Here's the drawing with two shaded views (mm, measured from the low corner). I have some questions. A direction names the side the tool comes from. Coordinates: 2 decimals unless noted, no trailing zeros. Write each loop counter-clockwise with the first axis right and the second up, starting at its lowest first coordinate (ties: lowest second). Pieces come first, ordered by that corner, then holes. Notation, with made-up numbers: (6.25, 34) - (12.25, 34) arc R22 ccw to (12.25, 60) - close; hole circle Ø4 at (-0.5, -3). An arc over 180 degrees is marked (long way). Answer in a Markdown table with one row per item. Add a question column.
Item 1: I'm going to push flat-ended pins straight in: pin 1 (1.8 mm diameter, centred on x = 3.5, y = 5.5, fed in from -Z); pin 2 (2 mm diameter, centred on x = 4.75, y = 4.75, fed in from -Z). Where does each tip first touch, or does it pass through?
Item 2: Imagine slicing it at B-B (y = 4.75). Please give me the cut outline in (x, z) (3 decimals).
Item 3: Imagine slicing it at D-D (z = 11.75). Please give me the cut outline in (x, y) (3 decimals), plus the area to 3 significant figures.
Item 4: Imagine slicing it at A-A (x = 4.75). Please give me the cut outline in (y, z).
Item 5: Imagine slicing it at C-C (x = 67.5). Please give me the cut outline in (y, z), plus the area to 3 significant figures.
Item 6: Which directions (+Z, -Z, +X, -X, +Y, -Y) give clear straight access to the entire face, cutting with the end or side of a thin tool? Please do the marked faces 1, 2 and 3.
Item 7: If I drill on probe 1 along Y at (x, z) = (4.75, 23); probe 2 along Y at (x, z) = (4.75, 11.75); probe 3 along X at (y, z) = (43.5, 2) (3 decimals), over which ranges is the centre line in solid material (lowest first)? Write a range as from..to.
Item 8: We'd pull the mould along X, two halves only. Please class the marked faces 4, 5 and 6: +X half, -X half, draft (parallel to the pull), parting line (faces both ways), or undercut.
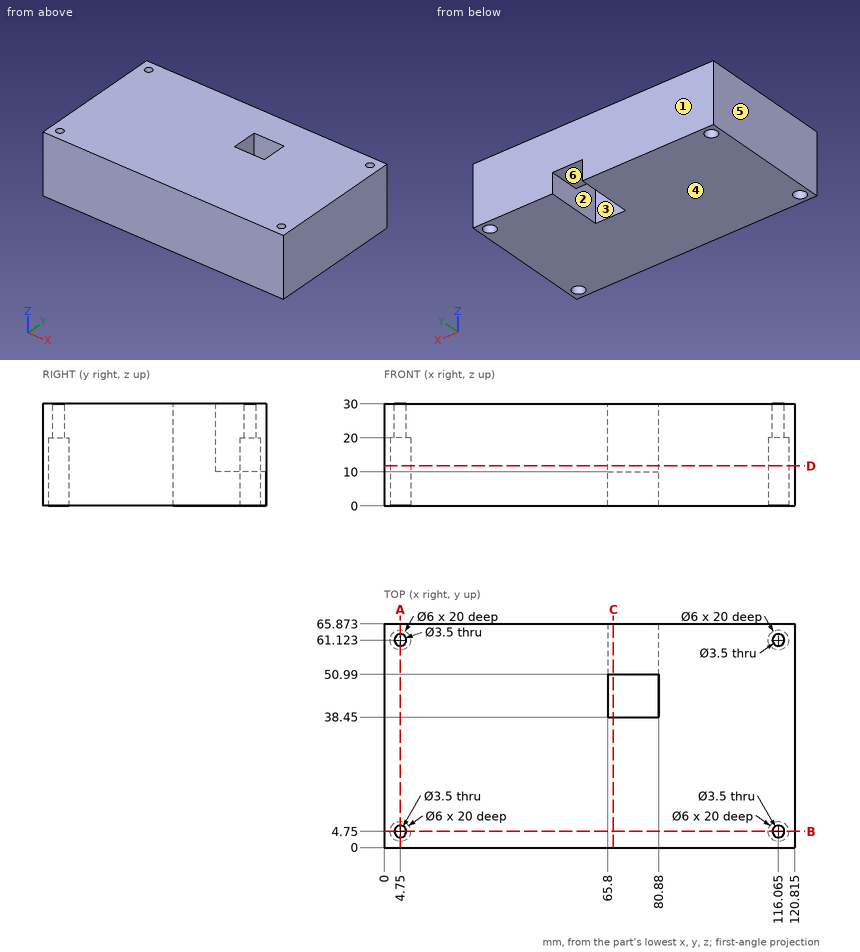
Here are the results:
| question | item | result |
|---|---|---|
| 1 | pin 1 | stops at z = 20 |
| 1 | pin 2 | passes through |
| 2 | outline | (0, 0) - (1.75, 0) - (1.75, 20) - (3, 20) - (3, 30) - (0, 30) - close; (6.5, 20) - (7.75, 20) - (7.75, 0) - (113.065, 0) - (113.065, 20) - (114.315, 20) - (114.315, 30) - (6.5, 30) - close; (117.815, 20) - (119.065, 20) - (119.065, 0) - (120.815, 0) - (120.815, 30) - (117.815, 30) - close |
| 3 | outline | (0, 0) - (120.815, 0) - (120.815, 65.873) - (0, 65.873) - close; hole circle Ø6 at (4.75, 4.75); hole circle Ø6 at (4.75, 61.123); hole (65.8, 38.45) - (80.88, 38.45) - (80.88, 50.99) - (65.8, 50.99) - close; hole circle Ø6 at (116.065, 4.75); hole circle Ø6 at (116.065, 61.123) |
| 3 | area | 7,660 mm2 |
| 4 | outline | (0, 0) - (1.75, 0) - (1.75, 20) - (3, 20) - (3, 30) - (0, 30) - close; (6.5, 20) - (7.75, 20) - (7.75, 0) - (58.12, 0) - (58.12, 20) - (59.37, 20) - (59.37, 30) - (6.5, 30) - close; (62.87, 20) - (64.12, 20) - (64.12, 0) - (65.87, 0) - (65.87, 30) - (62.87, 30) - close |
| 5 | outline | (0, 0) - (38.45, 0) - (38.45, 30) - (0, 30) - close; (50.99, 10) - (65.87, 10) - (65.87, 30) - (50.99, 30) - close |
| 5 | area | 1,450 mm2 |
| 6 | face 1 | +Z, -Z, +X, -X, +Y |
| 6 | face 2 | -Z |
| 6 | face 3 | +Z, -Z |
| 7 | probe 1 | y = 0..3, 6.5..59.37, 62.87..65.87 |
| 7 | probe 2 | y = 0..1.75, 7.75..58.12, 64.12..65.87 |
| 7 | probe 3 | x = 0..65.8, 80.88..120.815 |
| 8 | face 4 | draft |
| 8 | face 5 | -X half |
| 8 | face 6 | undercut |
